For this review, take the finished solid that the model builds, in its own axes (mm). A direction names the side the tool comes from. Round coordinates to 2 decimals unless told otherwise and drop trailing zeros. Write each loop counter-clockwise with the first axis right and the second up, starting at its lowest first coordinate (ties: lowest second). Pieces come first, ordered by that corner, then holes. Notation, with made-up numbers: (-2, 1.5) - (13, 1.5) arc R34 ccw to (13, 34.5) - close; hole circle Ø7 at (88, 72.25). An arc over 180 degrees is marked (long way). Answer in a Markdown table with one row per item. Add a question column.
from build123d import *

# Parameters (mm, degrees)
PAD_DEPTH        = 20
FILLET_R         = 15
HOLE_D           = 5
HOLE_CBORE_D     = 8
HOLE_CBORE_DEPTH = 3


with BuildPart() as part:
    # Sketch → Pad (new body, symmetric)
    with BuildSketch(Plane.XZ):
        Polygon((-15.515675, 80), (-15.515675, 0), (44.484325, 0), (44.484325, 10), (-0.515675, 10), (-0.515675, 80), align=None)
    extrude(amount=PAD_DEPTH, both=True)

    # Fillet
    fillet_edges = [part.edges().sort_by_distance(p)[0] for p in [
        (-8.015675, 20, 80),
        (-8.015675, -20, 80),
        (44.484325, 20, 5),
        (44.484325, -20, 5),
    ]]
    fillet(fillet_edges, radius=FILLET_R)

    # Hole (through all)
    with Locations(Plane.YZ):
        with Locations((-8, 65)):
            hole = CounterBoreHole(HOLE_D / 2, HOLE_CBORE_D / 2, HOLE_CBORE_DEPTH)

    # Mirrored: Hole across XZ
    add(hole.mirror(Plane.XZ), mode=Mode.SUBTRACT)


solid = part.part
Q1. Add section D-D on z = 17. State the section outline as (x, y) points.
Q2. Tool access review of faces 4 (the face through (-0.516, 0, 45)), 5 (the face through (-1.74, 8.867, 61.095)), 6 (the face through (-9.35, -10.31, 64.04)): name each direction out of +Z, -Z, +X, -X, +Y, -Y from which nothing blocks a thin tool from reaching the whole face with its end or side.
Q3. Add section A-A on x = -5.5. State the section outline as (y, z) points, then the cut area to 3 significant figures.
Q4. To check wall thickness, follow probe 1 along X at (y, z) = (-13.5, 25.5); probe 2 along Z at (x, y) = (-1.45, -8); probe 3 along Z at (x, y) = (1.5, -13). State the ranges of each line that lie inside material, in increasing order.
Q5. Draft analysis for pull direction Z (two halves, no side actions). For faces 1 (the face through (-15.516, 0, 41)), 2 (the face through (22, 0, 10)), 3 (the face through (-3, -10, 63)), state which applies: released by +Z, released by -Z, zero draft, split by the parting line, or undercut.
Q6. Insertion check: pin 1 Ø9 at (y, z) = (8, 65) entering from +X; pin 2 Ø6 at (y, z) = (8, 65) entering from -X; pin 3 Ø4 at (y, z) = (-9.5, 64) entering from +X; pin 4 Ø3 at (y, z) = (-8, 65) entering from +X. Each pin has a flat end and moves straight along its axis. Give the tip position at first contact, or say it passes through.
Q7. Add section B-B on z = 63.5. State the section outline as (x, y) points.
Q8. Add section C-C on y = -8. State the section outline as (x, z) points, then the cut area to 3 significant figures.
Answer sheet:
| question | item | result |
|---|---|---|
| 1 | outline | (-15.52, -20) - (-0.52, -20) - (-0.52, 20) - (-15.52, 20) - close |
| 2 | face 4 | +Z, +X, +Y, -Y |
| 2 | face 5 | +X |
| 2 | face 6 | +X, -X |
| 3 | outline | (-20, 0) - (20, 0) - (20, 65) arc R15 ccw to (5, 80) - (-5, 80) arc R15 ccw to (-20, 65) - close; hole circle Ø5 at (-8, 65); hole circle Ø5 at (8, 65) |
| 3 | area | 3,060 mm² |
| 4 | probe 1 | x = -15.52 to -0.52 |
| 4 | probe 2 | z = 0 to 61, 69 to 79.7 |
| 4 | probe 3 | z = 0 to 10 |
| 5 | face 1 | zero draft |
| 5 | face 2 | released by +Z |
| 5 | face 3 | undercut |
| 6 | pin 1 | stops at x = -0.52 |
| 6 | pin 2 | stops at x = -15.52 |
| 6 | pin 3 | stops at x = -3 |
| 6 | pin 4 | passes through |
| 7 | outline | (-15.52, -20) - (-0.52, -20) - (-0.52, -11.71) - (-3, -11.71) - (-3, -10) - (-15.52, -10) - close; (-15.52, -6) - (-3, -6) - (-3, -4.29) - (-0.52, -4.29) - (-0.52, 4.29) - (-3, 4.29) - (-3, 6) - (-15.52, 6) - close; (-15.52, 10) - (-3, 10) - (-3, 11.71) - (-0.52, 11.71) - (-0.52, 20) - (-15.52, 20) - close |
| 8 | outline | (-15.52, 0) - (44.18, 0) - (44.18, 10) - (-0.52, 10) - (-0.52, 61) - (-3, 61) - (-3, 62.5) - (-15.52, 62.5) - close; (-15.52, 67.5) - (-3, 67.5) - (-3, 69) - (-0.52, 69) - (-0.52, 79.7) - (-15.52, 79.7) - close |
| 8 | area | 1,560 mm² |
